For this review, take the finished solid that the model builds, in its own axes (mm). A direction names the side the tool comes from. Give positions to 0.01 mm unless a question says otherwise; leave off trailing zeros. Order: outer loops, then holes, each group sorted by start corner. A loop starts at its lowest first (then second) coordinate and runs counter-clockwise, first axis right, second up. Notation, with made-up numbers: (84.25, -17.75) - (127.25, -17.75) arc R31 ccw to (127.25, 18.25) - close; hole circle Ø2 at (51, 42.25). An arc over 180 degrees is marked (long way). Put each result on its own line as item: value. Start each with the question number.
```python
from build123d import *

# Parameters (mm, degrees)
SKETCH2_R               = 8.255
BOSS_EXTRUDE1_DEPTH     = 190.5
SKETCH3_W               = 19.05
SKETCH3_H               = 19.05
SKETCH3_W_2             = 2.54
SKETCH3_H_2             = 10.16
SKETCH6_R               = 19.05
SKETCH6_R_2             = 12.7
CUT_EXTRUDE1_DEPTH      = 2.54
SKETCH5_R               = 4.445
BOSS_EXTRUDE3_DEPTH     = 25.4
CIRPATTERN2_COUNT       = 5
MIRROR3_COPY_1_SKETCH_R = 4.445
MIRROR3_COPY_1_DEPTH    = 25.4
MIRROR3_COPY_2_SKETCH_R = 4.445
MIRROR3_COPY_2_DEPTH    = 25.4
MIRROR3_COPY_3_SKETCH_R = 4.445
MIRROR3_COPY_3_DEPTH    = 25.4
MIRROR3_COPY_4_SKETCH_R = 4.445
MIRROR3_COPY_4_DEPTH    = 25.4
SKETCH7_R               = 2.54
CUT_EXTRUDE2_DEPTH      = 206.628908418


with BuildPart() as part:
    # Sketch2 → Boss-Extrude1 (new, symmetric)
    with BuildSketch(Plane(origin=(0, 0, 0), x_dir=(0, 0, -1), z_dir=(1, 0, 0))):
        Circle(SKETCH2_R)
    extrude(amount=BOSS_EXTRUDE1_DEPTH, both=True)

    # Sketch3 → Revolve1 (revolve)
    with BuildSketch(Plane.XY, mode=Mode.PRIVATE) as revolve1_sk:
        with Locations((180.975, 17.78)):
            Rectangle(SKETCH3_W, SKETCH3_H)
        with Locations((100.33, 13.335)):
            Rectangle(SKETCH3_W_2, SKETCH3_H_2)
        with Locations((143.51, 13.335)):
            Rectangle(SKETCH3_W_2, SKETCH3_H_2)
        with Locations((-100.33, 13.335)):
            Rectangle(SKETCH3_W_2, SKETCH3_H_2)
        with Locations((-143.51, 13.335)):
            Rectangle(SKETCH3_W_2, SKETCH3_H_2)
        with Locations((-180.975, 17.78)):
            Rectangle(SKETCH3_W, SKETCH3_H)
    revolve(revolve1_sk.sketch.rotate(Axis((190.5, 0, 0), (-1, 0, 0)), 90), axis=Axis((190.5, 0, 0), (-1, 0, 0)))

    # Sketch6 → Cut-Extrude1 (cut)
    with BuildSketch(Plane.ZY.offset(190.5)):
        Circle(SKETCH6_R)
        Circle(SKETCH6_R_2, mode=Mode.SUBTRACT)
    cut_extrude1 = extrude(amount=-CUT_EXTRUDE1_DEPTH, mode=Mode.SUBTRACT)

    # Mirror2: Cut-Extrude1 across plane
    add(cut_extrude1.mirror(Plane(origin=(0, 0, 0), x_dir=(0, 0, 1), z_dir=(1, 0, 0))), mode=Mode.SUBTRACT)

    # Sketch5 → Boss-Extrude3 (add)
    with BuildSketch(Plane(origin=(0, 21.59, 0), x_dir=(1, 0, 0), z_dir=(0, 1, 0))):
        with Locations(Location((-180.975, 0, 0), (0, 0, 90))):
            Circle(SKETCH5_R)
    boss_extrude3 = extrude(amount=BOSS_EXTRUDE3_DEPTH)

    # CirPattern2: Boss-Extrude3 ×5 about axis
    cirpattern2_axis = Axis((0, 0, 0), (1, 0, 0))
    for i in range(1, CIRPATTERN2_COUNT):
        add(boss_extrude3.rotate(cirpattern2_axis, i * 360 / CIRPATTERN2_COUNT))

    # Mirror3: Boss-Extrude3 across plane
    add(boss_extrude3.mirror(Plane(origin=(0, 0, 0), x_dir=(0, 0, 1), z_dir=(1, 0, 0))))

    # Mirror3 copy 1 sketch → Mirror3 copy 1 (add)
    with BuildSketch(Plane(origin=(0, 6.671676909, 20.533310187), x_dir=(-1, 0, 0), z_dir=(0, 0.30901699437494745, 0.9510565162951535))):
        with Locations((-180.975, 0)):
            Circle(MIRROR3_COPY_1_SKETCH_R)
    extrude(amount=MIRROR3_COPY_1_DEPTH)

    # Mirror3 copy 2 sketch → Mirror3 copy 2 (add)
    with BuildSketch(Plane(origin=(0, -17.466676909, 12.690283597), x_dir=(-1, 0, 0), z_dir=(0, -0.8090169943749473, 0.5877852522924732))):
        with Locations((-180.975, 0)):
            Circle(MIRROR3_COPY_2_SKETCH_R)
    extrude(amount=MIRROR3_COPY_2_DEPTH)

    # Mirror3 copy 3 sketch → Mirror3 copy 3 (add)
    with BuildSketch(Plane(origin=(0, -17.466676909, -12.690283597), x_dir=(-1, 0, 0), z_dir=(0, -0.8090169943749476, -0.587785252292473))):
        with Locations((-180.975, 0)):
            Circle(MIRROR3_COPY_3_SKETCH_R)
    extrude(amount=MIRROR3_COPY_3_DEPTH)

    # Mirror3 copy 4 sketch → Mirror3 copy 4 (add)
    with BuildSketch(Plane(origin=(0, 6.671676909, -20.533310187), x_dir=(-1, 0, 0), z_dir=(0, 0.30901699437494723, -0.9510565162951536))):
        with Locations((-180.975, 0)):
            Circle(MIRROR3_COPY_4_SKETCH_R)
    extrude(amount=MIRROR3_COPY_4_DEPTH)

    # Sketch7 → Cut-Extrude2 (cut, through all)
    with BuildSketch(Plane(origin=(0, 21.59, 0), x_dir=(1, 0, 0), z_dir=(0, 1, 0))):
        with Locations(Location((-66.606224815, 0, 0), (0, 0, 270))):
            Circle(SKETCH7_R)
    extrude(amount=-CUT_EXTRUDE2_DEPTH, mode=Mode.SUBTRACT)


solid = part.part
```
1. Wall thickness on line 1 (Y direction, x = 189.8, z = 0) (3 decimals); line 2 (X direction, y = 21, z = -14); line 3 (X direction, y = -5, z = 0): over which ranges is each line inside the solid? List them lowest first. Write a range as from..to.
2. The part is to be moulded in two halves that separate along X. For faces 1 (the face through (190.5, -19, 6)), 2 (the face through (-171.45, -6, 6)), 3 (the face through (-190.5, 0, 0)), 4 (the face through (176.735, 10.108, 35.431)), say which applies: released by +X, released by -X, zero draft, split by the parting line, or undercut.
3. Add section A-A, the plane x = 32.5. Give the boundary of the cut face in (y, z) (3 decimals), then the cut area to 3 significant figures.
4. Tool access review of faces 5 (the face through (-176.636, 36.82, 0.964)), 6 (the face through (190.5, 0, 0)), 7 (the face through (-189.25, -12.4, -2.75)), 8 (the face through (181.04, 14.58, -44.67)), 9 (the face through (-144.78, 4, 8)): name each direction out of +Z, -Z, +X, -X, +Y, -Y from which nothing blocks a thin tool from reaching the whole face with its end or side.
5. Clearance check with flat-ended pins moving along their axes: pin 1 (6 mm diameter, centred on x = 82, z = -7, fed in from -Y); pin 2 (1 mm diameter, centred on x = -69, z = 7, fed in from -Y); pin 3 (4 mm diameter, centred on x = -144, z = 11.5, fed in from -Y). State where each tip first meets the part, or that it passes through.
Found:
1. line 1: y = -27.305..-19.05, -12.7..12.7, 19.05..27.305
1. line 2: x = -190.5..-171.45, 171.45..190.5
1. line 3: x = -190.5..-69.15, -64.07..190.5
2. face 1: released by +X
2. face 2: undercut
2. face 3: released by -X
2. face 4: undercut
3. outline: circle Ø16.51 at (0, 0)
3. area: 214 mm^2
4. face 5: +Y
4. face 6: +Z, -Z, +X, +Y, -Y
4. face 7: -X
4. face 8: -Z, +X, -X, +Y
4. face 9: none
5. pin 1: stops at y = -7.22
5. pin 2: stops at y = -5.09
5. pin 3: stops at y = -15.78
